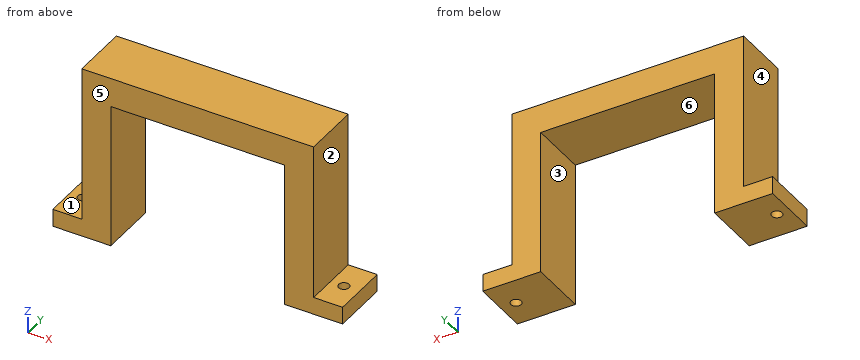
from build123d import *

# Parameters (mm, degrees)
F1_DEPTH = 25.4
F3_D     = 4.572
F5_D     = 4.572


with BuildPart() as f1:
    # F0 (on Front) → F1 (new body)
    with BuildSketch(Plane.XZ):
        Polygon((-45.351734, -7.193425), (-45.351734, -75.773425), (-58.051734, -75.773425), (-58.059905, -83.466448), (-32.651734, -83.466448), (-32.651734, -19.966448), (43.548266, -19.966448), (43.548266, -83.466448), (68.948266, -83.466448), (68.948266, -75.846448), (56.248266, -75.846448), (56.248266, -7.193425), align=None)
    extrude(amount=F1_DEPTH)

    # F3 (through all)
    with Locations(Plane.XY):
        with Locations((-52.30502, -12.795078)):
            Hole(F3_D / 2)

    # F5 (through all)
    with Locations(Plane.XY):
        with Locations((62.102944, -13.002886)):
            Hole(F5_D / 2)


solid = f1.part
The listing builds one solid part. Answer for the finished solid, in the listing's coordinates (mm). Face numbers are marked on the shaded views. A direction names the side the tool comes from. Give positions to 0.01 mm unless a question says otherwise; leave off trailing zeros. Loops run counter-clockwise (first coordinate to the right, second up) from the corner with the lowest first, then second, coordinate; pieces in that order, holes last. Notation, with made-up numbers: M 75.5,13 L 120.5,13 A33 cw 120.5,49 Z; hole C 32.25,16.25 d5. An arc over 180 degrees is marked long. Answer as CSV lines item,"result".
Item 1: The part is cut by section A-A (z = -77.5). Give the vertices of the cut face in (x, y), and give its area (3 significant figures).
Values follow:
outline,"M -58.05,-25.4 L -32.65,-25.4 L -32.65,0 L -58.05,0 Z; M 43.55,-25.4 L 68.95,-25.4 L 68.95,0 L 43.55,0 Z; hole C -52.31,-12.8 d4.57; hole C 62.1,-13 d4.57"
area,"1,260 mm^2"
Item 2: The part is cut by section B-B (z = -39). Give the vertices of the cut face in (x, y), and give its area (3 significant figures).
Values follow:
outline,"M -45.35,-25.4 L -32.65,-25.4 L -32.65,0 L -45.35,0 Z; M 43.55,-25.4 L 56.25,-25.4 L 56.25,0 L 43.55,0 Z"
area,"645 mm^2"
Item 3: Which of the six approach directions +Z, -Z, +X, -X, +Y, -Y give full straight-line access (tool end or side, diameter ignored) to the marked faces 1, 2 and 3?
Values follow:
face 1,"+Z, -X, +Y, -Y"
face 2,"+Z, +X, +Y, -Y"
face 3,"-Z, +Y, -Y"
Item 4: The part is cut by section C-C (y = -2). Give the vertices of the cut face in (x, z).
Values follow:
outline,"M -58.06,-83.47 L -32.65,-83.47 L -32.65,-19.97 L 43.55,-19.97 L 43.55,-83.47 L 68.95,-83.47 L 68.95,-75.85 L 56.25,-75.85 L 56.25,-7.19 L -45.35,-7.19 L -45.35,-75.77 L -58.05,-75.77 Z"
Item 5: The part is cut by section D-D (x = 37.5). Give the vertices of the cut face in (y, z).
Values follow:
outline,"M -25.4,-19.97 L 0,-19.97 L 0,-7.19 L -25.4,-7.19 Z"
Item 6: Straight lines are drawn through the part: line 1 along X through (y, z) = (-4.75, -60.5); line 2 along Z through (x, y) = (27, -20.75); line 3 along X through (y, z) = (-18.5, -13). For each, find the intervals that lie inside material, in ascending order. Write a range as [from, to].
Values follow:
line 1,"x = [-45.35, -32.65], [43.55, 56.25]"
line 2,"z = [-19.97, -7.19]"
line 3,"x = [-45.35, 56.25]"
Item 7: Given pin 1 Ø7.5 at (y, z) = (-17, -57) entering from -X; pin 2 Ø7.5 at (x, y) = (-52.31, -12.8) entering from +Z; pin 3 Ø10 at (x, z) = (9, -29) entering from +Y; pin 4 Ø1.5 at (y, z) = (-15.5, -42.5) entering from +X, each flat-ended and moving along its own axis, determine where each tip first touches the part or whether it passes through.
Values follow:
pin 1,"stops at x = -45.35"
pin 2,"stops at z = -75.77"
pin 3,"passes through"
pin 4,"stops at x = 56.25"
Item 8: The mould has two halves that part along X. Classify the marked faces 4, 5 and 6: released by +X, released by -X, zero draft, split by the parting line, or undercut.
Values follow:
face 4,"released by -X"
face 5,"zero draft"
face 6,"undercut"
